Answer from the drawing. Dimensions are ordinates in mm from the lowest x, y and z of the part. A direction names the side the tool comes from. Coordinates: 2 decimals unless noted, no trailing zeros. Write each loop counter-clockwise with the first axis right and the second up, starting at its lowest first coordinate (ties: lowest second). Pieces come first, ordered by that corner, then holes. Notation, with made-up numbers: (-17.75, 4) - (25.25, 4) arc R6 ccw to (25.25, 14) - close; hole circle Ø1 at (84, -33.75). An arc over 180 degrees is marked (long way). Answer as a JSON object with one key per item and string values. Group by question number.
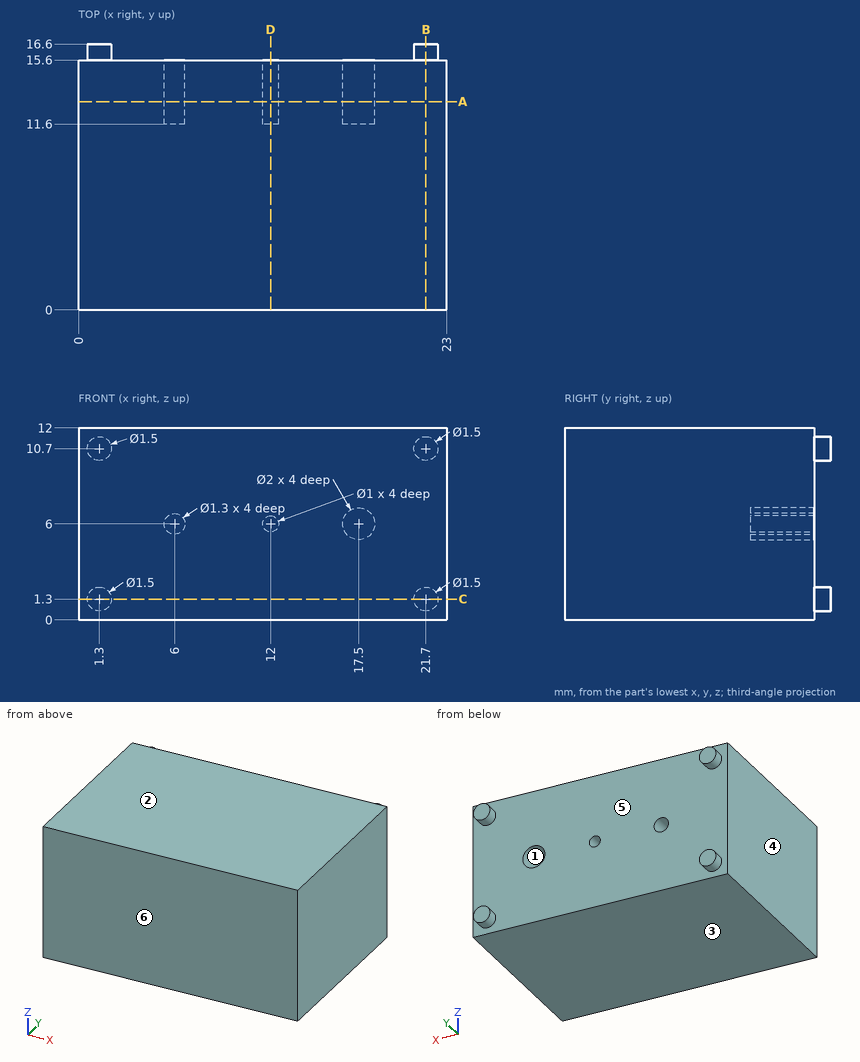
Q1. Section D-D on x = 12 is taken. Determine the outline of the cut face in (y, z), plus the area to 3 significant figures.
Q2. Consider L1, parallel to X at y = 13.1, z = 6; L2, parallel to Z at x = 6, y = 13.4; L3, parallel to Y at x = 20.75, z = 7.5. Determine where each line is inside the solid, lowest interval first. Write a range as from..to.
Q3. Section A-A on y = 13 is taken. Determine the outline of the cut face in (x, z).
Q4. For a pull along Z with two mould halves and no side action, classify the marked faces 1, 2, 3 and 4 as +Z half, -Z half, draft (parallel to the pull), parting line (faces both ways), or undercut.
Q5. Section C-C on z = 1.3 is taken. Determine the outline of the cut face in (x, y).
Q6. Flat-ended cylindrical pins translate along their axes: pin 1 Ø1 at (x, z) = (6, 6) entering from +Y; pin 2 Ø1.6 at (x, z) = (17.5, 5.5) entering from +Y. Find the tip coordinate at first contact, or state that the pin passes through.
Q7. A tool of negligible diameter and unlimited length cuts with its end or side. For the marked faces 5 and 6, from which of +Z, -Z, +X, -X, +Y, -Y can it reach the whole face along a straight path? Write none if from no direction.
Q8. Section B-B on x = 21.7 is taken. Determine the outline of the cut face in (y, z), plus the area to 3 significant figures.
Numbers:
{
 "1": {"outline": "(0, 0) - (15.6, 0) - (15.6, 5.5) - (11.6, 5.5) - (11.6, 6.5) - (15.6, 6.5) - (15.6, 12) - (0, 12) - close", "area": "183 mm²"},
 "2": {"L1": "x = 0..5.35, 6.65..11.5, 12.5..16.5, 18.5..23", "L2": "z = 0..5.35, 6.65..12", "L3": "y = 0..15.6"},
 "3": {"outline": "(0, 0) - (23, 0) - (23, 12) - (0, 12) - close; hole circle Ø1.3 at (6, 6); hole circle Ø1 at (12, 6); hole circle Ø2 at (17.5, 6)"},
 "4": {"face 1": "undercut", "face 2": "+Z half", "face 3": "-Z half", "face 4": "draft"},
 "5": {"outline": "(0, 0) - (23, 0) - (23, 15.6) - (22.45, 15.6) - (22.45, 16.6) - (20.95, 16.6) - (20.95, 15.6) - (2.05, 15.6) - (2.05, 16.6) - (0.55, 16.6) - (0.55, 15.6) - (0, 15.6) - close"},
 "6": {"pin 1": "stops at y = 11.6", "pin 2": "stops at y = 15.6"},
 "7": {"face 5": "+Y", "face 6": "+Z, -Z, +X, -X, -Y"},
 "8": {"outline": "(0, 0) - (15.6, 0) - (15.6, 0.55) - (16.6, 0.55) - (16.6, 2.05) - (15.6, 2.05) - (15.6, 9.95) - (16.6, 9.95) - (16.6, 11.45) - (15.6, 11.45) - (15.6, 12) - (0, 12) - close", "area": "190 mm²"}
}
